Work out the finished part from the listing and answer in its coordinate system (mm). Face numbers are marked on the shaded views. A direction names the side the tool comes from. Coordinates: 2 decimals unless noted, no trailing zeros. Write each loop counter-clockwise with the first axis right and the second up, starting at its lowest first coordinate (ties: lowest second). Pieces come first, ordered by that corner, then holes. Notation, with made-up numbers: (45, -18.75) - (95, -18.75) arc R24 ccw to (95, -0.75) - close; hole circle Ø1 at (39, 1). An arc over 180 degrees is marked (long way). One line per item, written item: value.
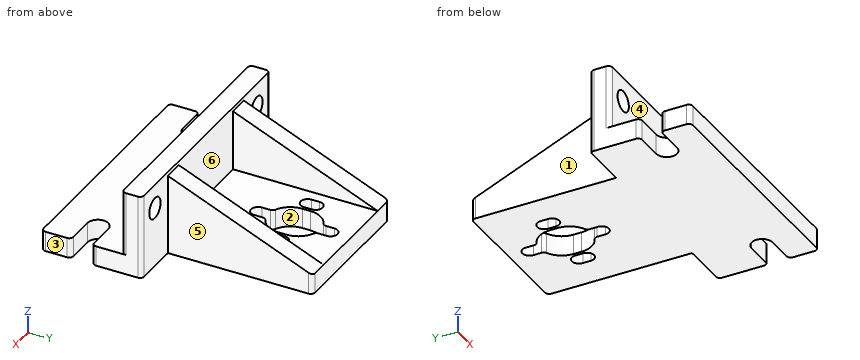
Autodesk Fusion 360 part; units mm, degrees
sketch "スケッチ1" plane through (0, 0, 0) normal (0, 0, 1) x (1, 0, 0)
  line L0 (-17.5, 0) -> (-17.5, 36)
  line L1 (-17.5, 36) -> (17.5, 36)
  line L2 (17.5, 36) -> (17.5, 0)
  line L3 (-29.5, 0) -> (29.5, 0)
  line L4 (29.5, 0) -> (29.5, -25)
  line L5 (29.5, -25) -> (-29.5, -25)
  line L6 (-29.5, -25) -> (-29.5, 0)
  line L7 (-29.5, -5) -> (29.5, -5)
  line L8 (-12.5, 0) -> (-12.5, 36)
  line L9 (12.5, 0) -> (12.5, 36)
  circle A0 centre (22, -15) radius 2.6
  circle A1 centre (-22, -15) radius 2.6
  line L10 (29.5, -12.4) -> (22, -12.4)
  line L11 (29.5, -17.6) -> (22, -17.6)
  line L12 (-29.5, -12.4) -> (-22, -12.4)
  line L13 (-29.5, -17.6) -> (-22, -17.6)
  circle A2 centre (0, 23) radius 5.5
  circle A3 centre (0, 21) radius 5.5
  circle A4 centre (0, 31) radius 1.75
  circle A5 centre (0, 13) radius 1.75
  line L14 (0, 36) -> (0, 0) construction
  line L15 (1.75, 31) -> (1.75, 28.2142)
  line L16 (-1.75, 31) -> (-1.75, 28.2142)
  line L17 (1.75, 13) -> (1.75, 15.7858)
  line L18 (-1.75, 13) -> (-1.75, 15.7858)
  line L19 (5.5, 23) -> (5.5, 21)
  line L20 (-8, 23) -> (-8, 21)
  circle A6 centre (-8, 23) radius 1.75
  circle A7 centre (-8, 21) radius 1.75
  line L21 (-6.25, 21) -> (-6.25, 23)
  line L22 (-9.75, 21) -> (-9.75, 23)
  circle A8 centre (8, 23) radius 1.75
  line L23 (6.25, 21) -> (6.25, 23)
  circle A9 centre (8, 21) radius 1.75
  line L24 (9.75, 21) -> (9.75, 23)
  line L25 (-5.5, 23) -> (-5.5, 21)
  dimension "d1" = 36
  dimension "d2" = 25
  dimension "d3" = 5
  dimension "d4" = 35
  dimension "d5" = 59
  dimension "d6" = 17.5
  dimension "d7" = 5
  dimension "d8" = 5
  dimension "d9" = 5.2
  dimension "d10" = 5.2
  dimension "d11" = 7.5
  dimension "d12" = 7.5
  dimension "d13" = 10
  dimension "d14" = 10
  dimension "d15" = 11
  dimension "d16" = 11
  dimension "d17" = 3.5
  dimension "d18" = 3.5
  dimension "d19" = 5
  dimension "d20" = 18
  dimension "d21" = 2
  dimension "d22" = 8
  dimension "d23" = 2
  dimension "d24" = 3.5
  dimension "d25" = 3.5
  dimension "d26" = 8
  dimension "d27" = 8
extrude "押し出し1" add sketch "スケッチ1" along normal blind 5 contours L3 L4 L6 L7 | L1 L3 L8 L9 | L4 L5 L6 L7 A0 A1 L10 L11 L12 L13
extrude "押し出し2" add sketch "スケッチ1" along normal blind 21 contours L3 L4 L6 L7
extrude "押し出し3" add sketch "スケッチ1" along normal blind 20 contours L0 L1 L3 L8 | L1 L2 L3 L9
chamfer "面取り1" distance 36 distance2 15 2 edges at (-15, 36, 20) (15, 36, 20) measured on face at (-15.8333, 24, 20) measured on face at (14.1667, 12, 20)
hole "穴1" at (23.5, -5, 15) direction (0, 1, 0) diameter 5.2 depth 6 tip angle 118
hole "穴2" at (-23.5, -5, 15) direction (0, 1, 0) diameter 5.2 depth 6 tip angle 118
fillet "フィレット1" radius 1 12 edges at (29.5, -25, 2.5) (29.5, -17.6, 2.5) (29.5, -12.4, 2.5) (29.5, -5, 13) (29.5, 0, 10.5) (17.5, 36, 2.5) (-17.5, 36, 2.5) (-29.5, 0, 10.5) (-29.5, -5, 13) (-29.5, -25, 2.5) (-29.5, -17.6, 2.5) (-29.5, -12.4, 2.5)
fillet "フィレット2" radius 1 4 edges at (1.75, 28.2142, 2.5) (1.75, 15.7858, 2.5) (-1.75, 15.7858, 2.5) (-1.75, 28.2142, 2.5)
equation "d6 = d4 / 2"
Item 1: Determine the mould class of the marked faces 1, 2 and 3 for opening direction X: +X half, -X half, draft (parallel to the pull), parting line (faces both ways), or undercut.
Evaluation:
face 1: -X half
face 2: undercut
face 3: +X half
Item 2: Section D-D, the plane z = 8 is taken. Determine the outline of the cut face in (x, y).
Evaluation:
outline: (-29.5, -4) arc R1 ccw to (-28.5, -5) - (28.5, -5) arc R1 ccw to (29.5, -4) - (29.5, -1) arc R1 ccw to (28.5, 0) - (17.5, 0) - (17.5, 28.81) - (12.5, 28.81) - (12.5, 0) - (-12.5, 0) - (-12.5, 28.81) - (-17.5, 28.81) - (-17.5, 0) - (-28.5, 0) arc R1 ccw to (-29.5, -1) - close
Item 3: Section B-B, the plane x = 23.5 is taken. Determine the outline of the cut face in (y, z).
Evaluation:
outline: (-25, 0) - (-17.6, 0) - (-17.6, 5) - (-25, 5) - close; (-12.4, 0) - (0, 0) - (0, 12.4) - (-5, 12.4) - (-5, 5) - (-12.4, 5) - close; (-5, 17.6) - (0, 17.6) - (0, 21) - (-5, 21) - close
Item 4: Which of the six approach directions +Z, -Z, +X, -X, +Y, -Y give full straight-line access (tool end or side, diameter ignored) to the marked faces 4, 5 and 6?
Evaluation:
face 4: +Z, +X, -X, -Y
face 5: +Z, -Z, +X, +Y
face 6: +Z, +Y
Item 5: Section C-C, the plane y = 26.5 is taken. Determine the outline of the cut face in (x, z).
Evaluation:
outline: (-17.5, 0) - (-4.24, 0) - (-4.24, 5) - (-12.5, 5) - (-12.5, 8.96) - (-17.5, 8.96) - close; (4.24, 0) - (17.5, 0) - (17.5, 8.96) - (12.5, 8.96) - (12.5, 5) - (4.24, 5) - close
Item 6: Given pin 1 (1.7 mm diameter, centred on y = 14.5, z = 2.5, fed in from -X); pin 2 (1.5 mm diameter, centred on y = 18, z = 10.5, fed in from +X); pin 3 (17 mm diameter, centred on x = 0, y = -19, fed in from +Z), each flat-ended and moving along its own axis, determine where each tip first touches the part or whether it passes through.
Evaluation:
pin 1: stops at x = -17.5
pin 2: stops at x = 17.5
pin 3: stops at z = 5
Item 7: Consider probe 1 along X at (y, z) = (-1.4, 15); probe 2 along Y at (x, z) = (26.5, 3); probe 3 along X at (y, z) = (21, 6.25). Determine where each line is inside the solid, lowest interval first.
Evaluation:
probe 1: x = -29.5 to -26.1, -20.9 to 20.9, 26.1 to 29.5
probe 2: y = -25 to -17.6, -12.4 to 0
probe 3: x = -17.5 to -12.5, 12.5 to 17.5
Item 8: Section A-A, the plane x = 0 is taken. Determine the outline of the cut face in (y, z), then the cut area to 4 significant figures.
Evaluation:
outline: (-25, 0) - (11.25, 0) - (11.25, 5) - (0, 5) - (0, 21) - (-5, 21) - (-5, 5) - (-25, 5) - close; (32.75, 0) - (36, 0) - (36, 5) - (32.75, 5) - close
area: 277.5 mm2
